For this review, take the finished solid that the model builds, in its own axes (mm). A direction names the side the tool comes from. Coordinates: 2 decimals unless noted, no trailing zeros. Write each loop counter-clockwise with the first axis right and the second up, starting at its lowest first coordinate (ties: lowest second). Pieces come first, ordered by that corner, then holes. Notation, with made-up numbers: M 29,34.25 L 38,34.25 A21 ccw 38,66.25 Z; hole C 16.25,62 d3. An arc over 180 degrees is marked long. Return JSON: item names as keys, results as strings.
```python
from build123d import *

# Parameters (mm, degrees)
F1_DEPTH = 279.4
F2_T     = -18.1428571429
F3_R     = 18.5632222349
F4_DEPTH = 25.4


with BuildPart() as f1:
    # F0 (on Top) → F1 (new body)
    with BuildSketch(Plane.XY):
        Polygon((43.678151575, 8.2475193234), (14.6965145353, 41.950148516), (-28.9816370398, 33.7026291926), (-43.678151575, -8.2475193234), (-14.6965145353, -41.950148516), (28.9816370398, -33.7026291926), align=None)
    extrude(amount=F1_DEPTH)

    # F2
    f2_openings = [f1.faces().sort_by_distance(p)[0] for p in [
        (0, 0, 279.4),
    ]]
    offset(amount=F2_T, openings=f2_openings)

    # F3 (on face) → F4 (cut)
    with BuildSketch(Plane(origin=(36.3298943074, -12.7275549346, 0), x_dir=(0.3306302483, 0.9437603716, 0), z_dir=(0.9437603716, -0.3306302483, 0))):
        with Locations((0, 154.4703543186)):
            Circle(F3_R)
    extrude(amount=-F4_DEPTH, mode=Mode.SUBTRACT)


solid = f1.part
```
1. Wall thickness on L1, parallel to Z at x = 26, y = -8; L2, parallel to Z at x = -19, y = 3.5; L3, parallel to X at y = -6, z = 42: over which ranges is each line inside the solid? List them lowest first. Write a range as from..to.
Checks:
{"L1": "0..135.94, 173..279.4", "L2": "0..18.14", "L3": "-42.89..-21.68, 19.46..38.69"}
2. Draft analysis for pull direction Z (two halves, no side actions). For faces 3 (the face through (21.04, -27.02, 155.29)), 4 (the face through (15.54, 13.14, 146.94)), 5 (the face through (-1, 1, 0)), state which applies: +Z half, -Z half, draft (parallel to the pull), parting line (faces both ways), or undercut.
Checks:
{"face 3": "undercut", "face 4": "draft", "face 5": "-Z half"}
3. We need section B-B (x = 1). State the section outline as (y, z) points, plus the area to 3 significant figures.
Checks:
{"outline": "M -38.99,0 L 39.36,0 L 39.36,279.4 L 20.9,279.4 L 20.9,18.14 L -20.52,18.14 L -20.52,279.4 L -38.99,279.4 Z", "area": "11,100 mm2"}
4. For faces 1 (the face through (19.153, -6.884, 78.267)), 2 (the face through (6.837, -37.884, 137.744)), list the 3-axis set-ups (+Z, -Z, +X, -X, +Y, -Y) from which the entire face can be reached by the end or side of a thin tool; tool diameter is ignored.
Checks:
{"face 1": "+Z", "face 2": "+Z, -Z, +X, -Y"}
5. We need section C-C (y = 27). State the section outline as (x, z) points.
Checks:
{"outline": "M -31.33,0 L 27.55,0 L 27.55,279.4 L -31.33,279.4 Z"}
6. We need section A-A (z = 250). State the section outline as (x, y) points, plus the area to 3 significant figures.
Checks:
{"outline": "M -43.68,-8.25 L -14.7,-41.95 L 28.98,-33.7 L 43.68,8.25 L 14.7,41.95 L -28.98,33.7 Z; hole M -23.09,-4.36 L -7.77,-22.18 L 15.32,-17.82 L 23.09,4.36 L 7.77,22.18 L -15.32,17.82 Z", "area": "3,700 mm2"}
7. Clearance check with flat-ended pins moving along their axes: pin 1 Ø2 at (y, z) = (3, 64) entering from -X; pin 2 Ø12 at (x, z) = (31, 172) entering from +Y; pin 3 Ø3 at (y, z) = (-7.5, 207) entering from +X. State where each tip first meets the part, or that it passes through.
Checks:
{"pin 1": "x = -40.09", "pin 2": "y = 29.97", "pin 3": "x = 38.69"}
